Could you check a few things on this model? Use its own coordinates, in mm. A direction names the side the tool comes from. Coordinates: 2 decimals unless noted, no trailing zeros. Order: outer loops, then holes, each group sorted by start corner. A loop starts at its lowest first (then second) coordinate and runs counter-clockwise, first axis right, second up. Notation, with made-up numbers: (54.25, 1) -> (88.25, 1) arc R19 cw to (88.25, 27) -> close; hole circle Ø5 at (10, 48). An arc over 180 degrees is marked (long way). Use a Markdown table: item, result. Add a question column.
1) If I drill on L1, parallel to Z at x = 34, y = -12.7; L2, parallel to Y at x = 58, z = 2.5; L3, parallel to Z at x = 64.5, y = -19.5, over which ranges is the centre line in solid material (lowest first)? Write a range as [from, to].
2) If we section it at C-C (z = 29.5): Write out the boundary of the cut face in (x, y).
3) If we section it at A-A (y = -12.7): Write out the boundary of the cut face in (x, z).
4) If we section it at D-D (x = 27.5): Write out the boundary of the cut face in (y, z).
5) Thinking about a two-plate mould opening in Z: for faces 1 (the cylindrical face through (38.278, -6.643, 33.657)), 2 (the flat face through (19, -10, 12.7)), 3 (the cylindrical face through (4.294, -22.328, 6.439)), which applies, +Z half, -Z half, draft (parallel to the pull), parting line (faces both ways), or undercut?
6) Which directions (+Z, -Z, +X, -X, +Y, -Y) give clear straight access to the entire face, cutting with the end or side of a thin tool? Please do faces 4 (the cylindrical face through (38.28, -3.32, 40.4)), 5 (the flat face through (50.8, -13, 25)), 6 (the flat face through (25.4, -13, 25)).
7) Will these pins go through, and if not, where does the flat tip stop? pin 1 Ø12.5 at (y, z) = (-8.5, 26.5) entering from -X; pin 2 Ø12 at (x, z) = (50.5, 39) entering from -Y; pin 3 Ø7.5 at (x, y) = (17, -10.5) entering from +Z.
8) If we section it at B-B (x = 63.5): Write out the boundary of the cut face in (y, z).
```python
from build123d import *

# Parameters (mm, degrees)
F1_DEPTH = 25.4
F2_R     = 6.35
F3_DEPTH = 25.4
F4_R     = 6.35
F5_DEPTH = 12.7
F6_R     = 6.35
F7_DEPTH = 12.7


with BuildPart() as f1:
    # F0 (on Front) → F1 (new body)
    with BuildSketch(Plane.XZ):
        Polygon((0, 12.7), (0, 0), (76.2, 0), (76.2, 12.7), (50.8, 12.7), (50.8, 44.45), (25.4, 44.45), (25.4, 12.7), align=None)
    extrude(amount=F1_DEPTH)

    # F2 (on face) → F3 (cut)
    with BuildSketch(Plane.YZ.offset(50.8)):
        with Locations((-12.7, 31.75)):
            Circle(F2_R)
        with BuildLine():
            ThreePointArc((-11.1926886687, 44.45), (-3.231292005, 40.303582652), (0, 31.9288966496))
            Line((0, 31.9288966496), (0, 44.45))
            Line((0, 44.45), (-11.1926886687, 44.45))
        make_face()
        with BuildLine():
            ThreePointArc((-25.4, 31.9288966496), (-22.168707995, 40.303582652), (-14.2073113313, 44.45))
            Line((-14.2073113313, 44.45), (-25.4, 44.45))
            Line((-25.4, 44.45), (-25.4, 31.9288966496))
        make_face()
    extrude(amount=-F3_DEPTH, mode=Mode.SUBTRACT)

    # F4 (on face) → F5 (cut)
    with BuildSketch(Plane.XY.offset(12.7)):
        with Locations((63.5, -12.7)):
            Circle(F4_R)
        with BuildLine():
            ThreePointArc((64.3000455197, 0), (71.8337545006, -2.7749851952), (76.2, -9.512433828))
            Line((76.2, -9.512433828), (76.2, 0))
            Line((76.2, 0), (64.3000455197, 0))
        make_face()
        with BuildLine():
            ThreePointArc((76.2, -15.887566172), (71.8337545006, -22.6250148048), (64.3000455197, -25.4))
            Line((64.3000455197, -25.4), (76.2, -25.4))
            Line((76.2, -25.4), (76.2, -15.887566172))
        make_face()
    extrude(amount=-F5_DEPTH, mode=Mode.SUBTRACT)

    # F6 (on face) → F7 (cut)
    with BuildSketch(Plane.XY.offset(12.7)):
        with Locations((12.7, -12.7)):
            Circle(F6_R)
        with BuildLine():
            ThreePointArc((0, -10.9318505954), (4.1984404998, -3.1550374284), (12.4538305262, 0))
            Line((12.4538305262, 0), (0, 0))
            Line((0, 0), (0, -10.9318505954))
        make_face()
        with BuildLine():
            ThreePointArc((12.4538305262, -25.4), (4.1984404998, -22.2449625716), (0, -14.4681494046))
            Line((0, -14.4681494046), (0, -25.4))
            Line((0, -25.4), (12.4538305262, -25.4))
        make_face()
    extrude(amount=-F7_DEPTH, mode=Mode.SUBTRACT)


solid = f1.part
```
Answer sheet:
| question | item | result |
|---|---|---|
| 1 | L1 | [0, 25.4], [38.1, 44.45] |
| 1 | L2 | [-25.4, -15.87], [-9.53, 0] |
| 1 | L3 | [0, 12.7] |
| 2 | outline | (25.4, -25.4) -> (50.8, -25.4) -> (50.8, -18.64) -> (25.4, -18.64) -> close; (25.4, -6.76) -> (50.8, -6.76) -> (50.8, 0) -> (25.4, 0) -> close |
| 3 | outline | (0, 0) -> (6.35, 0) -> (6.35, 12.7) -> (0, 12.7) -> close; (19.05, 0) -> (57.15, 0) -> (57.15, 12.7) -> (50.8, 12.7) -> (50.8, 25.4) -> (25.4, 25.4) -> (25.4, 12.7) -> (19.05, 12.7) -> close; (25.4, 38.1) -> (50.8, 38.1) -> (50.8, 44.45) -> (25.4, 44.45) -> close; (69.85, 0) -> (76.2, 0) -> (76.2, 12.7) -> (69.85, 12.7) -> close |
| 4 | outline | (-25.4, 0) -> (0, 0) -> (0, 31.93) arc R12.7 ccw to (-11.19, 44.45) -> (-14.21, 44.45) arc R12.7 ccw to (-25.4, 31.93) -> close; hole circle Ø12.7 at (-12.7, 31.75) |
| 5 | face 1 | undercut |
| 5 | face 2 | +Z half |
| 5 | face 3 | draft |
| 6 | face 4 | +Z, +X, -X, +Y |
| 6 | face 5 | +Z, +X, +Y, -Y |
| 6 | face 6 | +Z, -X, +Y, -Y |
| 7 | pin 1 | x = 25.4 |
| 7 | pin 2 | y = -25.35 |
| 7 | pin 3 | z = 12.7 |
| 8 | outline | (-25.4, 0) -> (-19.05, 0) -> (-19.05, 12.7) -> (-25.4, 12.7) -> close; (-6.35, 0) -> (0, 0) -> (0, 12.7) -> (-6.35, 12.7) -> close |
